The model under review builds one solid part; all positions refer to its coordinate system, in mm. A direction names the side the tool comes from. Give positions to 0.01 mm unless a question says otherwise; leave off trailing zeros. Order: outer loops, then holes, each group sorted by start corner. A loop starts at its lowest first (then second) coordinate and runs counter-clockwise, first axis right, second up. Notation, with made-up numbers: M 56,-14.75 L 104,-14.75 A22 ccw 104,12.25 Z; hole C 51.5,-33.75 d8. An arc over 180 degrees is marked long. One line per question, with ' | ' between items. Start each with the question number.
1. Wall thickness on L1, parallel to X at y = 16.9, z = 2.7; L2, parallel to Y at x = 30, z = 1; L3, parallel to Y at x = 119, z = 1.1: over which ranges is each line inside the solid? List them lowest first.
2. We need section C-C on x = 29. Write out the cut boundary in (y, z), then the cut area to 3 significant figures.
3. We need section B-B on x = 58.5. Write out the cut boundary in (y, z), then the cut area to 3 significant figures.
4. Insertion check: P1, Ø1.1, axis at y = -17, z = 1.5, coming from the +X side; P2, Ø1, axis at x = 60.5, z = 0.5, coming from the -Y side; P3, Ø4.5, axis at x = 137.13, y = 3.5, coming from the -Z side; P4, Ø2, axis at y = 9.5, z = 3, coming from the +X side. Each pin has a flat end and moves straight along its axis. Give the tip position at first contact, or say it passes through.
5. We need section A-A on x = 104.6. Write out the cut boundary in (y, z).
6. For faces 5 (the face through (59, -20, 2)), 6 (the face through (52, -15.8, 2)), 7 (the face through (58, 1, 0)), list the 3-axis set-ups (+Z, -Z, +X, -X, +Y, -Y) from which the entire face can be reached by the end or side of a thin tool; tool diameter is ignored.
7. The part is to be moulded in two halves that separate along X. For faces 1 (the face through (99, 18, 2)), 2 (the face through (58, 1, 4)), 3 (the face through (-24.078, -12.802, 1.972)), 4 (the face through (45.732, 0.664, 1.972)), say which applies: +X half, -X half, draft (parallel to the pull), parting line (faces both ways), or undercut.
8. We need section D-D on z = 3.15. Count the separate pieces of the cut face and the enclosed holes in it, then the cut area to 3 significant figures.
```python
from build123d import *

# Parameters (mm, degrees)
SKETCH_1_R      = 4.25
SKETCH_1_R_2    = 8.75
SKETCH_1_R_3    = 2
SKETCH_1_R_4    = 1.5
SKETCH_1_R_5    = 3.5
SKETCH_1_W      = 4.2
SKETCH_1_H      = 2.2
EXTRUDE_1_DEPTH = 4


with BuildPart() as part:
    # 草图1 → 凸台-拉伸1 (new body)
    with BuildSketch(Plane.XY):
        with BuildLine():
            Line((-1, 20), (124.064295006, 20))
            ThreePointArc((124.064295006, 20), (144.064295006, 0), (124.064295006, -20))
            Line((124.064295006, -20), (10.014533743, -20))
            Line((10.014533743, -20), (-8.201544029, -20))
            Line((-8.201544029, -20), (-21.728077025, -28.201893958))
            ThreePointArc((-21.728077025, -28.201893958), (-29.496403282, -28.496403282), (-29.201893958, -20.728077025))
            Line((-29.201893958, -20.728077025), (-18.809358134, -4.651044611))
            Line((-18.809358134, -4.651044611), (-19.264777912, 8.14848991))
            ThreePointArc((-19.264777912, 8.14848991), (-11.886464114, 16.777511708), (-1, 20))
        make_face()
        with Locations((-1, 0)):
            Circle(SKETCH_1_R, mode=Mode.SUBTRACT)
        with Locations((124.064295006, 0)):
            Circle(SKETCH_1_R_2, mode=Mode.SUBTRACT)
        with Locations((114.497140256, 9.567154749)):
            Circle(SKETCH_1_R_3, mode=Mode.SUBTRACT)
        with Locations((137.133271435, 3.50182168)):
            Circle(SKETCH_1_R_3, mode=Mode.SUBTRACT)
        with Locations((120.562473325, -13.06897643)):
            Circle(SKETCH_1_R_3, mode=Mode.SUBTRACT)
        with Locations(Location((29, 16.9, 0), (0, 0, 180))):
            Circle(SKETCH_1_R_4, mode=Mode.SUBTRACT)
        with Locations(Location((104.6, 16.9, 0), (0, 0, 180))):
            Circle(SKETCH_1_R_4, mode=Mode.SUBTRACT)
        with Locations((-25.748737342, -24.748737342)):
            Circle(SKETCH_1_R_5, mode=Mode.SUBTRACT)
        with Locations((11.106307295, 12.106307295)):
            Circle(SKETCH_1_R_4, mode=Mode.SUBTRACT)
        with Locations(Location((58.5, -16.9, 0), (0, 0, 180))):
            Circle(SKETCH_1_R_4, mode=Mode.SUBTRACT)
        with BuildLine():
            Line((32.894135197, 8.030421477), (100.819514517, -9.118068433))
            ThreePointArc((100.819514517, -9.118068433), (101.678794604, -8.937407044), (102.064295006, -8.14848991))
            Line((102.064295006, -8.14848991), (102.064295006, 9))
            ThreePointArc((102.064295006, 9), (101.771401787, 9.707106781), (101.064295006, 10))
            Line((101.064295006, 10), (33.138915685, 10))
            ThreePointArc((33.138915685, 10), (32.146550197, 9.123331822), (32.894135197, 8.030421477))
        make_face(mode=Mode.SUBTRACT)
        with BuildLine():
            Line((12.244780488, 9.118068433), (80.170159809, -8.030421477))
            ThreePointArc((80.170159809, -8.030421477), (80.917744808, -9.123331822), (79.925379321, -10))
            Line((79.925379321, -10), (12, -10))
            ThreePointArc((12, -10), (11.292893219, -9.707106781), (11, -9))
            Line((11, -9), (11, 8.14848991))
            ThreePointArc((11, 8.14848991), (11.385500402, 8.937407044), (12.244780488, 9.118068433))
        make_face(mode=Mode.SUBTRACT)
        with Locations((35, 16.9)):
            Rectangle(SKETCH_1_W, SKETCH_1_H, mode=Mode.SUBTRACT)
        with Locations((98.6, 16.9)):
            Rectangle(SKETCH_1_W, SKETCH_1_H, mode=Mode.SUBTRACT)
        with Locations((52.5, -16.9)):
            Rectangle(SKETCH_1_W, SKETCH_1_H, mode=Mode.SUBTRACT)
    extrude(amount=EXTRUDE_1_DEPTH)


solid = part.part
```
Entries:
1) L1: x = -11.7 to 27.5, 30.5 to 32.9, 37.1 to 96.5, 100.7 to 103.1, 106.1 to 134.76 | L2: y = -20 to -10, 4.64 to 15.78, 18.02 to 20 | L3: y = -20 to -14.32, -11.82 to -7.14, 7.14 to 20
2) outline: M -20,0 L -10,0 L -10,4 L -20,4 Z; M 4.89,0 L 15.4,0 L 15.4,4 L 4.89,4 Z; M 18.4,0 L 20,0 L 20,4 L 18.4,4 Z | area: 88.4 mm^2
3) outline: M -20,0 L -18.4,0 L -18.4,4 L -20,4 Z; M -15.4,0 L -10,0 L -10,4 L -15.4,4 Z; M -2.56,0 L 1.57,0 L 1.57,4 L -2.56,4 Z; M 10,0 L 20,0 L 20,4 L 10,4 Z | area: 84.5 mm^2
4) P1: stops at x = 135.44 | P2: stops at y = -20 | P3: stops at z = 0 | P4: stops at x = 142.17
5) outline: M -20,0 L 15.4,0 L 15.4,4 L -20,4 Z; M 18.4,0 L 20,0 L 20,4 L 18.4,4 Z
6) face 5: +Z, -Z, +X, -Y | face 6: +Z, -Z | face 7: -Z, +X, -X, +Y, -Y
7) face 1: undercut | face 2: draft | face 3: -X half | face 4: undercut
8) separate pieces: 1 | enclosed holes: 15 | area: 4,590 mm^2
